The listing builds one solid part. Answer for the finished solid, in the listing's coordinates (mm). A direction names the side the tool comes from. Round coordinates to 2 decimals unless told otherwise and drop trailing zeros. Loops run counter-clockwise (first coordinate to the right, second up) from the corner with the lowest first, then second, coordinate; pieces in that order, holes last. Notation, with made-up numbers: (18, 81) -> (37, 81) arc R25 ccw to (37, 102) -> close; hole circle Ø8 at (2.25, 44.25). An arc over 180 degrees is marked (long way). One line per question, with ' | ' between items.
from build123d import *
from OCP.BRepFilletAPI import BRepFilletAPI_MakeChamfer

# Parameters (mm, degrees)
CHANFREIN1_SIZE            = 0.5
CHANFREIN1_SIZE2           = 0.288675135
ESQUISSE2_W                = 1.25
ESQUISSE2_H                = 6
TROU_TARAUD_M31_AT_2_COUNT = 2
TROU_TARAUD_M31_AT_2_PITCH = 10


with BuildPart() as part:
    # Esquisse1 → Révolution1 (revolve)
    with BuildSketch(Plane.XY, mode=Mode.PRIVATE) as r_volution1_sk:
        Polygon((0, 3), (0, 6), (16, 6), (16, 2), (8, 2), (8, 3), align=None)
    revolve(r_volution1_sk.sketch.rotate(Axis((0, 0, 0), (1, 0, 0)), 90), axis=Axis((0, 0, 0), (1, 0, 0)))

    # Chanfrein1: one chamfer whose edges measure the first distance from different faces: ONE call of the kernel's chamfer builder (chamfer() names one face for all edges)
    chanfrein1_edges_1 = [part.edges().sort_by_distance(p)[0] for p in [
        (16, 0, -2),
    ]]
    chanfrein1_side_1 = [part.faces().sort_by_distance(p)[0] for p in [
        (12, 0, -2),
    ]]
    chanfrein1_edges_2 = [part.edges().sort_by_distance(p)[0] for p in [
        (16, 0, -6),
    ]]
    chanfrein1_side_2 = [part.faces().sort_by_distance(p)[0] for p in [
        (16, 0, -5.830294373),
    ]]
    chanfrein1_edges_3 = [part.edges().sort_by_distance(p)[0] for p in [
        (0, 0, -6),
    ]]
    chanfrein1_side_3 = [part.faces().sort_by_distance(p)[0] for p in [
        (8, 0, -6),
    ]]
    chanfrein1_edges_4 = [part.edges().sort_by_distance(p)[0] for p in [
        (0, 0, -3),
    ]]
    chanfrein1_side_4 = [part.faces().sort_by_distance(p)[0] for p in [
        (0, 0, -3.169705627),
    ]]
    chanfrein1 = BRepFilletAPI_MakeChamfer(part.part.solid().wrapped)
    for e in chanfrein1_edges_1:
        chanfrein1.Add(CHANFREIN1_SIZE, CHANFREIN1_SIZE2, e.wrapped, chanfrein1_side_1[0].wrapped)  # the first distance lies on this face
    for e in chanfrein1_edges_2:
        chanfrein1.Add(CHANFREIN1_SIZE, CHANFREIN1_SIZE2, e.wrapped, chanfrein1_side_2[0].wrapped)  # the first distance lies on this face
    for e in chanfrein1_edges_3:
        chanfrein1.Add(CHANFREIN1_SIZE, CHANFREIN1_SIZE2, e.wrapped, chanfrein1_side_3[0].wrapped)  # the first distance lies on this face
    for e in chanfrein1_edges_4:
        chanfrein1.Add(CHANFREIN1_SIZE, CHANFREIN1_SIZE2, e.wrapped, chanfrein1_side_4[0].wrapped)  # the first distance lies on this face
    add(Compound.cast(chanfrein1.Shape()), mode=Mode.REPLACE)

    # Esquisse2 → Trou taraudé M31 (revolve, cut)
    with BuildSketch(Plane.YZ.offset(3)):
        with Locations((0.625, 3)):
            Rectangle(ESQUISSE2_W, ESQUISSE2_H)
    trou_taraud_m31 = revolve(axis=Axis((3, 0, -6.35), (0, 0, 1)), mode=Mode.SUBTRACT)

    # Trou taraudé M31 at 2: Trou taraudé M31 ×2
    with Locations(*[(i * TROU_TARAUD_M31_AT_2_PITCH, 0, 0) for i in range(1, TROU_TARAUD_M31_AT_2_COUNT)]):
        add(trou_taraud_m31, mode=Mode.SUBTRACT)


solid = part.part
Q1. For faces 1 (the face through (4, 0, -3)), 2 (the face through (12.95, -1.25, 3.81)), 3 (the face through (0, 4, 0)), determine the directions among +Z, -Z, +X, -X, +Y, -Y from which every point of the face is accessible in a straight line to the end or side of a thin tool.
Numbers:
face 1: -X | face 2: +Z | face 3: +Z, -Z, -X, +Y, -Y
Q2. Given pin 1 Ø4 at (x, y) = (10.5, -3.5) entering from +Z; pin 2 Ø5 at (y, z) = (0.5, 0.5) entering from -X; pin 3 Ø4.5 at (y, z) = (0, 0) entering from -X, each flat-ended and moving along its own axis, determine where each tip first touches the part or whether it passes through.
Numbers:
pin 1: z = 5.81 | pin 2: x = 0.17 | pin 3: x = 8
Q3. For a pull along Z with two mould halves and no side action, classify faces 4 (the face through (8.212, -1.802, 5.723)), 5 (the face through (8, 2, -1)), 6 (the face through (1.76, -0.16, 4.39)) as pulls with the +Z half, pulls with the -Z half, needs draft (parallel to the pull), parting line crosses it, or undercut.
Numbers:
face 4: parting line crosses it | face 5: undercut | face 6: needs draft
Q4. A cutting plane is placed at D-D on x = 5.5. Give the vertices of the cut face in (y, z), plus the area to 3 significant figures.
Numbers:
outline: circle Ø12 at (0, 0); hole circle Ø6 at (0, 0) | area: 84.8 mm^2
Q5. A cutting plane is placed at B-B on z = 0. Give the vertices of the cut face in (x, y).
Numbers:
outline: (0, -5.71) -> (0.5, -6) -> (15.71, -6) -> (16, -5.5) -> (16, -2.29) -> (15.5, -2) -> (8, -2) -> (8, -3) -> (0.29, -3) -> (0, -3.5) -> close; (0, 3.5) -> (0.29, 3) -> (8, 3) -> (8, 2) -> (15.5, 2) -> (16, 2.29) -> (16, 5.5) -> (15.71, 6) -> (0.5, 6) -> (0, 5.71) -> close
Q6. A cutting plane is placed at C-C on x = 14.5. Give the vertices of the cut face in (y, z).
Numbers:
outline: circle Ø12 at (0, 0); hole circle Ø4 at (0, 0)
Q7. Find the intervals of material crossed by line 1 (Y direction, x = 13, z = 0); line 2 (Z direction, x = 3.75, y = 0); line 3 (Z direction, x = 13, y = 0), in increasing order. Write a range as from..to.
Numbers:
line 1: -6..-2, 2..6 | line 2: -6..-3 | line 3: -6..-2
Q8. A cutting plane is placed at A-A on y = 0. Give the vertices of the cut face in (x, z), plus the area to 3 significant figures.
Numbers:
outline: (0, -5.71) -> (0.5, -6) -> (15.71, -6) -> (16, -5.5) -> (16, -2.29) -> (15.5, -2) -> (8, -2) -> (8, -3) -> (0.29, -3) -> (0, -3.5) -> close; (0, 3.5) -> (0.29, 3) -> (1.75, 3) -> (1.75, 6) -> (0.5, 6) -> (0, 5.71) -> close; (4.25, 3) -> (8, 3) -> (8, 2) -> (11.75, 2) -> (11.75, 6) -> (4.25, 6) -> close; (14.25, 2) -> (15.5, 2) -> (16, 2.29) -> (16, 5.5) -> (15.71, 6) -> (14.25, 6) -> close | area: 93.9 mm^2
